```python
from build123d import *

# Parameters (mm, degrees)
CUT_EXTRUDE1_DEPTH      = 32.163141952
CUT_EXTRUDE1_DEPTH_BACK = 32.163141952
FILLET1_R               = 0.5


# Read off the part's stored shape, not the designer's step: Revolve2
with BuildPart() as part:
    # Revolve2 outline → Revolve2 (revolve)
    with BuildSketch(Plane.YX):
        Polygon((7.75, 28.118346614), (0, 28.118346614), (0, 7.618346614), (6.35, 7.618346614), (9.5, 14.118346614), (9.5, 21.118346614), (7.75, 21.118346614), align=None)
    revolve(axis=Axis((0, 0, 0), (1, 0, 0)))

    # Sketch3 → Cut-Extrude1 (cut, two sides: drawn at the far end of the back side and taken through both)
    with BuildSketch(Plane(origin=(0, 0, 0), x_dir=(1, 0, 0), z_dir=(0, 1, 0)).offset(-CUT_EXTRUDE1_DEPTH_BACK)):
        with BuildLine():
            Line((7.618346614, 6.35), (7.618346614, -6.35))
            ThreePointArc((7.618346614, -6.35), (9.046260231, 0), (7.618346614, 6.35))
        make_face()
    extrude(amount=CUT_EXTRUDE1_DEPTH + CUT_EXTRUDE1_DEPTH_BACK, mode=Mode.SUBTRACT)

    # Fillet1
    fillet1_edges = [part.edges().sort_by_distance(p)[0] for p in [
        (28.118346614, -7.75, 0),
    ]]
    fillet(fillet1_edges, radius=FILLET1_R)


solid = part.part
```
For this review, take the finished solid that the model builds, in its own axes (mm). A direction names the side the tool comes from. Round coordinates to 2 decimals unless told otherwise and drop trailing zeros. Write each loop counter-clockwise with the first axis right and the second up, starting at its lowest first coordinate (ties: lowest second). Pieces come first, ordered by that corner, then holes. Notation, with made-up numbers: (54.5, -15.5) -> (80.5, -15.5) arc R24 ccw to (80.5, 19.5) -> close; hole circle Ø3 at (-36.75, 50). An arc over 180 degrees is marked (long way). One line per question, with ' | ' between items. Start each with the question number.
1) Add section C-C (x = 18). Write out the cut boundary in (y, z), and give its area (3 significant figures).
2) Add section B-B (x = 26). Write out the cut boundary in (y, z), and give its area (3 significant figures).
3) For pin 1 Ø4 at (x, y) = (18, -5.5) entering from +Z; pin 2 Ø5 at (x, z) = (23.5, -2) entering from -Y; pin 3 Ø8 at (x, y) = (18.5, -7) entering from +Z; pin 4 Ø6 at (x, y) = (23, 0) entering from -Z, all flat-tipped, find the tip position at first contact; note any pin that passes through.
4) Mouldability with a two-part tool opening along Z and no side actions: class faces 3 (the cylindrical face through (17.67, 4.38, -8.43)), 4 (the cylindrical face through (9.046, -0.099, 0.092)), 5 (the flat face through (21.118, -8, 0)) as +Z half, -Z half, draft (parallel to the pull), parting line (faces both ways), or undercut.
5) Machinability: for faces 1 (the cylindrical face through (24.414, -1.009, 7.684)), 2 (the conical face through (8.02, -1.42, -6.39)), which of the approach directions +Z, -Z, +X, -X, +Y, -Y give a long, thin tool a straight path to every point of the face, cutting with its end or side? Answer none if there is none.
6) Add section A-A (z = 0). Write out the cut boundary in (x, y), and give its area (3 significant figures).
7) Wall thickness on line 1 along Y through (x, z) = (23.25, 0.25); line 2 along Y through (x, z) = (14, 7); line 3 along X through (y, z) = (-3.5, 7): over which ranges is each line inside the solid? List them lowest first.
Reported:
1) outline: circle Ø19 at (0, 0) | area: 284 mm²
2) outline: circle Ø15.5 at (0, 0) | area: 189 mm²
3) pin 1: stops at z = 8.83 | pin 2: stops at y = -9.42 | pin 3: stops at z = 9.01 | pin 4: stops at z = -9.5
4) face 3: parting line | face 4: undercut | face 5: draft
5) face 1: +X | face 2: -X
6) outline: (9.05, -7.04) -> (14.12, -9.5) -> (21.12, -9.5) -> (21.12, -7.75) -> (27.62, -7.75) arc R0.5 ccw to (28.12, -7.25) -> (28.12, 7.25) arc R0.5 ccw to (27.62, 7.75) -> (21.12, 7.75) -> (21.12, 9.5) -> (14.12, 9.5) -> (9.05, 7.04) -> close | area: 325 mm²
7) line 1: y = -7.75 to 7.75 | line 2: y = -6.34 to 6.34 | line 3: x = 10.66 to 21.12
